Can you work these out from the drawing? Everything is in mm from the part's minimum corner. A direction names the side the tool comes from. Give positions to 0.01 mm unless a question says otherwise; leave off trailing zeros. Write each loop counter-clockwise with the first axis right and the second up, starting at its lowest first coordinate (ties: lowest second). Pieces come first, ordered by that corner, then holes. Notation, with made-up numbers: (8, -22.75) -> (49, -22.75) arc R24 ccw to (49, -3.75) -> close; hole circle Ø3 at (27, 60.25). An arc over 180 degrees is marked (long way). Return JSON: item names as keys, results as strings.
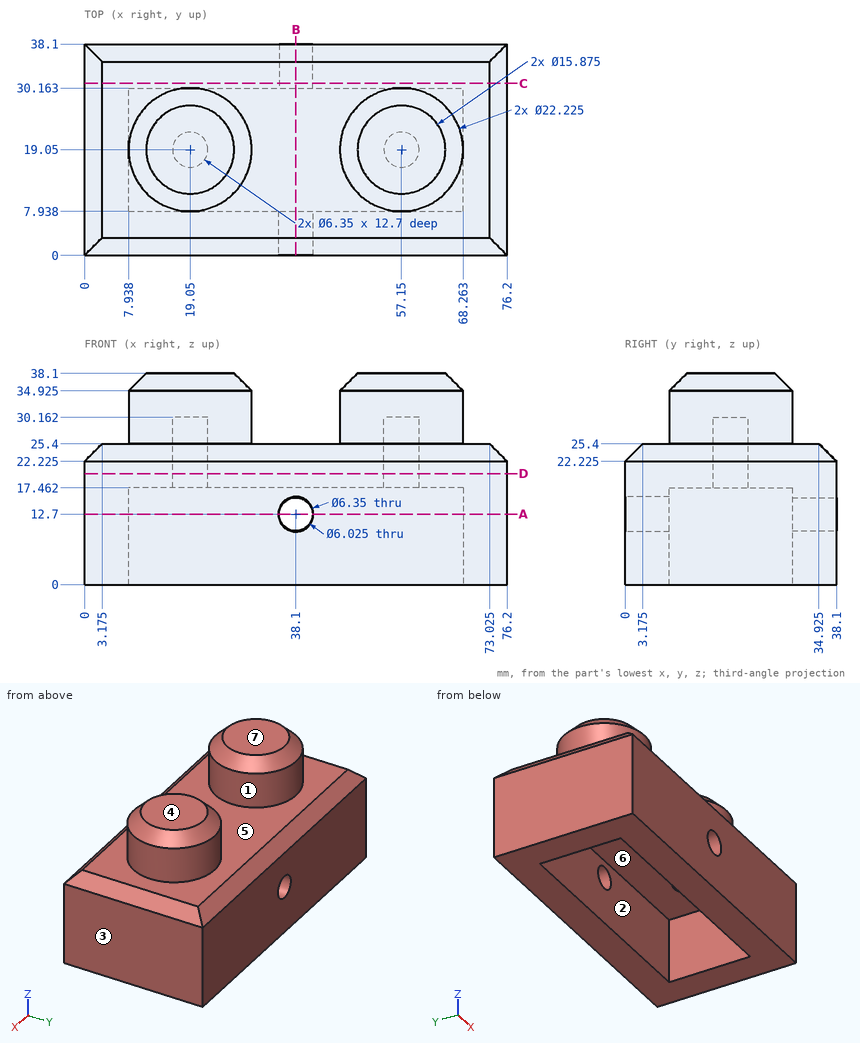
1. Suppose I cut it at D-D, the plane z = 20. Count the separate pieces of the cut face and the enclosed holes in it, and give its area (3 significant figures).
Taken from the geometry:
{"separate pieces": "1", "enclosed holes": "2", "area": "2,840 mm²"}
2. Which directions (+Z, -Z, +X, -X, +Y, -Y) give clear straight access to the entire face, cutting with the end or side of a thin tool? Please do the marked faces 5, 6 and 7.
Taken from the geometry:
{"face 5": "+Z", "face 6": "-Z", "face 7": "+Z, +X, -X, +Y, -Y"}
3. Suppose I cut it at B-B, the plane x = 38.1. List the corners of the cut face in (y, z) for me (1 decimal), and give its area (3 significant figures).
Taken from the geometry:
{"outline": "(0, 0) -> (7.9, 0) -> (7.9, 9.5) -> (0, 9.5) -> close; (0, 15.9) -> (7.9, 15.9) -> (7.9, 17.5) -> (30.2, 17.5) -> (30.2, 15.7) -> (38.1, 15.7) -> (38.1, 22.2) -> (34.9, 25.4) -> (3.2, 25.4) -> (0, 22.2) -> close; (30.2, 0) -> (38.1, 0) -> (38.1, 9.7) -> (30.2, 9.7) -> close", "area": "471 mm²"}
4. For pin 1 Ø12 at (x, z) = (64.5, 32) entering from -Y; pin 2 Ø1.9 at (x, y) = (19.5, 18.5) entering from -Z; pin 3 Ø1 at (y, z) = (24, 23) entering from -X (1 decimal), each with a flat end and sliding along its axis, tell me the tip position at first contact or that it passes through.
Taken from the geometry:
{"pin 1": "stops at y = 8.02", "pin 2": "stops at z = 30.16", "pin 3": "stops at x = 0.3"}
5. If I drill on line 1 (X direction, y = 19, z = 20) (1 decimal); line 2 (X direction, y = 26.5, z = 15.5); line 3 (Y direction, x = 34.5, z = 14), over which ranges is the centre line in solid material (lowest first)? Write a range as [from, to].
Taken from the geometry:
{"line 1": "x = [0, 15.9], [22.2, 54], [60.3, 76.2]", "line 2": "x = [0, 7.94], [68.26, 76.2]", "line 3": "y = [0, 7.94], [30.16, 38.1]"}
6. If we mould it in two halves opening along X, with no side actions, what happens to the marked faces 1, 2, 3 and 4? For each: released by +X, released by -X, zero draft, split by the parting line, or undercut.
Taken from the geometry:
{"face 1": "undercut", "face 2": "undercut", "face 3": "released by +X", "face 4": "zero draft"}
7. Suppose I cut it at A-A, the plane z = 12.7. List the corners of the cut face in (x, y) for me (1 decimal).
Taken from the geometry:
{"outline": "(0, 0) -> (34.9, 0) -> (34.9, 7.9) -> (7.9, 7.9) -> (7.9, 30.2) -> (35.1, 30.2) -> (35.1, 38.1) -> (0, 38.1) -> close; (41.1, 30.2) -> (68.3, 30.2) -> (68.3, 7.9) -> (41.3, 7.9) -> (41.3, 0) -> (76.2, 0) -> (76.2, 38.1) -> (41.1, 38.1) -> close"}
8. Suppose I cut it at C-C, the plane y = 31. List the corners of the cut face in (x, z) for me (1 decimal), and give its area (3 significant figures).
Taken from the geometry:
{"outline": "(0, 0) -> (76.2, 0) -> (76.2, 22.2) -> (73, 25.4) -> (3.2, 25.4) -> (0, 22.2) -> close; hole circle Ø6 at (38.1, 12.7)", "area": "1,900 mm²"}
